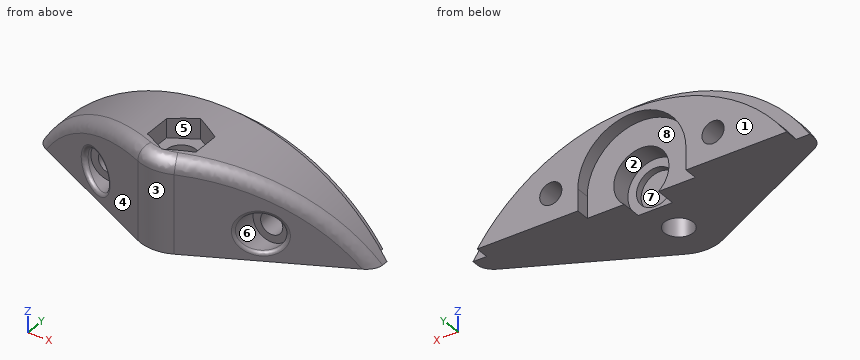
Autodesk Inventor part; units mm, degrees
ref_plane "Work Plane1" through (0, 0, 0) normal (0, 1, 0) x (-1, 0, 0)
ref_plane "Work Plane2" through (0, 11.1125, 46.99) normal (0, 0, 1) x (1, 0, 0)
ref_plane "YZ Plane" through (0, 0, 0) normal (1, 0, 0) x (0, 1, 0)
sketch "Sketch1" plane through (0, 0, 0) normal (0, 0, 1) x (1, 0, 0)
  line L0 (0, 0) -> (46.99, 0)
  line L1 (46.99, 0) -> (46.99, 22.225)
  line L2 (46.99, 22.225) -> (0, 22.225)
  line L3 (0, 22.225) -> (0, 0)
  line L4 (0, 22.225) -> (44.323, 22.225)
  line L5 (44.323, 22.225) -> (44.323, 25.4254)
  line L6 (44.323, 25.4254) -> (0, 25.4254)
  line L7 (0, 25.4254) -> (0, 22.225)
  circle A0 centre (0, 9.525) radius 9.525
  circle A1 centre (0, 9.525) radius 3.175
  line L8 (46.99, 22.225) -> (4.2364, 0.994)
  line L9 (0, 0) -> (-46.99, 0)
  line L10 (-46.99, 0) -> (-46.99, 22.225)
  line L11 (-46.99, 22.225) -> (0, 22.225)
  line L12 (0, 22.225) -> (0, 0)
  line L13 (-46.99, 22.225) -> (-4.2364, 0.994)
  dimension "d2" = 44.323
  dimension "d3" = 3.2004
  dimension "d5" = 6.35
  dimension "d7" = 6.35
  dimension "d67" = 12.7
  dimension "d119" = 46.99
revolve "Revolution1" add sketch "Sketch1" angle 180 about axis through (0, 22.225, 0) along (0, -1, 0) picked at (0.942, 16.8272) picked at (0.9535, 9.9842) contours A0 L8 L1 L0 | L3 A1 A0 | L3 A1 | A0 L3 L2 L8 | L2 L7 L6 L5
sketch "Sketch2" plane through (0, 0, 0) normal (1, 0, 0) x (0, 1, 0)
  line L0 (0, 0) -> (22.225, 0)
  line L1 (25.4254, 44.323) -> (25.4254, 0)
  line L2 (0, 0) -> (25.4254, 0)
  line L3 (25.4254, 0) -> (25.4254, 25.4)
  line L4 (25.4254, 25.4) -> (0, 25.4)
  line L5 (0, 25.4) -> (0, 0)
  dimension "d10" = 25.4
extrude "Extrusion1" cut sketch "Sketch2" along normal through all both and the other way through all
extrude "Extrusion2" cut sketch "Sketch1" along normal through all contours A0 L8 L1 L0 | L9 L10 L13 A0
ref_plane "Work Plane1" through (0, 0, 0) normal (0, 1, 0) x (-1, 0, 0)
sketch "Sketch9" plane through (0, 0, 0) normal (0, 1, 0) x (-1, 0, 0)
  line L0 (-19.05, 31.75) -> (0, 0) construction
  line L1 (0, 0) -> (19.05, 31.75) construction
  dimension "d46" = 31.75
  dimension "d47" = 38.1
hole "Hole1" at (19.05, 0, 31.75) at (-19.05, 0, 31.75) direction (0, 1, 0) diameter 5.207 end through all counterbore diameter 8.7313 counterbore depth 12.7
ref_plane "Work Plane2" through (0, 11.1125, 46.99) normal (0, 0, 1) x (1, 0, 0)
sketch "Sketch10" plane through (0, 11.1125, 46.99) normal (0, 0, 1) x (1, 0, 0)
  arc A0 (-4.2364, -10.1185) -> (4.2364, -10.1185) centre (0, -1.5875) ccw
  point P0 (0, -11.1125)
hole "Hole2" at (0, 9.525, 46.99) direction (0, 0, -1) diameter 6.7564 end through all
fillet "Fillet1" radius 0.7937 4 edges at (19.05, 8.3503, 36.1156) (-19.05, 8.3503, 36.1156) (-3.3781, 9.4995, 46.8684) (3.3781, 9.4966, 46.8684)
fillet "Fillet2" radius 3.175 4 edges at (2.2299, 0.2647, 46.9371) (-2.2284, 0.2643, 46.9371) (-24.3604, 10.9873, 40.1825) (24.3604, 10.9873, 40.1825)
sketch "Sketch12" plane through (0, 0, 0) normal (1, 0, 0) x (0, 1, 0)
  line L0 (12.9032, 25.4) -> (6.1468, 25.4)
  line L1 (22.225, 17.78) -> (22.225, 30.48)
  line L2 (43.3764, 30.48) -> (22.225, 30.48)
  line L3 (43.3764, 30.48) -> (43.3764, 17.78)
  line L4 (43.3764, 17.78) -> (22.225, 17.78)
  point P0 (0, 0)
  point P1 (9.525, 25.4)
  dimension "d108" = 12.7
  dimension "d111" = 30.48
  dimension "d120" = 12.7
revolve "Revolution2" cut sketch "Sketch12" angle 360 about axis through (0, 43.3764, 30.48) along (0, -1, 0)
sketch "Sketch13" plane through (0, 11.1125, 46.99) normal (0, 0, 1) x (1, 0, 0)
  circle A0 centre (0, -1.5875) radius 3.3782
  line L0 (0, 4.975) -> (5.6832, 1.6937)
  line L1 (5.6832, 1.6937) -> (5.6832, -4.8687)
  line L2 (5.6832, -4.8687) -> (0, -8.15)
  line L3 (0, -8.15) -> (-5.6833, -4.8687)
  line L4 (-5.6833, -4.8687) -> (-5.6832, 1.6937)
  line L5 (-5.6832, 1.6937) -> (0, 4.975)
  point P0 (0, -11.1125)
  dimension "d91" = 11.3665
extrude "Extrusion8" cut sketch "Sketch13" against normal blind 4.7625
sketch "Sketch14" plane through (39.5335, 22.225, 25.4) normal (0, 0, -1) x (-1, 0, 0)
  line L0 (26.8335, 0) -> (26.8335, 3.2004)
  line L1 (52.2335, 0) -> (52.2335, 3.2004)
  line L2 (52.2335, 0) -> (26.8335, 0)
  line L3 (26.8335, 3.2004) -> (52.2335, 3.2004)
  point P0 (39.5335, -22.225)
  point P1 (51.1733, 0)
  point P2 (27.8938, 0)
  point P3 (27.8938, 3.2004)
  point P4 (51.1733, 3.2004)
extrude "Extrusion9" cut sketch "Sketch14" against normal blind 5.08
sketch "Sketch15" plane through (0, 22.225, 30.48) normal (0, 1, 0) x (1, 0, 0)
  circle A0 centre (0, 0) radius 6.477
  arc A1 (-12.7, 0) -> (12.7, 0) centre (0, 0) ccw
  point P0 (0, 30.48)
  dimension "d98" = 12.954
hole "Hole5" at (0, 22.225, 30.48) direction (0, -1, 0) diameter 8.89 depth 6.35 counterbore diameter 12.954 counterbore depth 4.7752
properties part number "WheelBracketHead" material "ABS Plastic"
Geometry check sheet. Reference: the model listing, model coordinates, mm. Face numbers are marked on the shaded views. A direction names the side the tool comes from. Round coordinates to 2 decimals unless told otherwise and drop trailing zeros. Loops run counter-clockwise (first coordinate to the right, second up) from the corner with the lowest first, then second, coordinate; pieces in that order, holes last. Notation, with made-up numbers: (80, -39) -> (84, -39) arc R26 ccw to (84, -24) -> close; hole circle Ø4 at (60.5, 8). An arc over 180 degrees is marked (long way). Use a Markdown table: item, result.
(1) Mould release check, pull along X, two halves, no side actions. Record for the marked faces 1, 2, 3 and 4: released by +X, released by -X, zero draft, split by the parting line, or undercut.
Calculated:
| item | result |
|---|---|
| face 1 | zero draft |
| face 2 | undercut |
| face 3 | split by the parting line |
| face 4 | released by -X |
(2) Go/stop test with flat-tipped pins: P1, Ø1.5, axis at x = -7.5, z = 38, coming from the -Y side; P2, Ø1.5, axis at y = 5.5, z = 34.5, coming from the +X side; P3, Ø2, axis at y = 14.5, z = 35.5, coming from the -X side. Record where each tip stops, or that it passes through.
Calculated:
| item | result |
|---|---|
| P1 | y = 2.24 |
| P2 | x = 14.82 |
| P3 | x = -30.95 |
(3) Sectioned sample at B-B (z = 31.75). Give the number of separate pieces and of enclosed holes in the cut face, then the cut area to 3 significant figures.
Calculated:
| item | result |
|---|---|
| separate pieces | 3 |
| enclosed holes | 1 |
| area | 813 mm² |
(4) Set-up check for the marked faces 5, 6, 7 and 8: record each of +Z, -Z, +X, -X, +Y, -Y from which the full face is reachable in a straight line by a thin tool's end or side.
Calculated:
| item | result |
|---|---|
| face 5 | +Z |
| face 6 | -Y |
| face 7 | +Y |
| face 8 | -Z, +Y |
(5) Scan lines: probe 1 along X at (y, z) = (13.25, 29.75); probe 2 along X at (y, z) = (11.75, 35.5); probe 3 along X at (y, z) = (13, 30.25). Record each from-to range of solid material in increasing order.
Calculated:
| item | result |
|---|---|
| probe 1 | -28.92 to -20.72, -17.38 to 17.38, 20.72 to 28.92 |
| probe 2 | -25.9 to -21.29, -16.81 to -2.54, 2.54 to 16.81, 21.29 to 25.9 |
| probe 3 | -28.41 to -21.18, -16.92 to 16.92, 21.18 to 28.41 |
(6) Sectioned sample at A-A (y = 23.5). Enter the section's corners in (x, z).
Calculated:
| item | result |
|---|---|
| outline | (-36.32, 25.4) -> (-12.7, 25.4) -> (-12.7, 30.48) arc R12.7 cw to (12.7, 30.48) -> (12.7, 25.4) -> (36.32, 25.4) arc R44.32 ccw to start; hole circle Ø5.21 at (-19.05, 31.75); hole circle Ø5.21 at (19.05, 31.75) |
